The listing builds one solid part. Answer for the finished solid, in the listing's coordinates (mm). Face numbers are marked on the shaded views. A direction names the side the tool comes from. Give positions to 0.01 mm unless a question says otherwise; leave off trailing zeros. Order: outer loops, then holes, each group sorted by start corner. A loop starts at its lowest first (then second) coordinate and runs counter-clockwise, first axis right, second up.
```python
from build123d import *

# Parameters (mm, degrees)
BOSS_EXTRUDE1_DEPTH = 25.4
SKETCH3_R           = 4.05
CUT_EXTRUDE1_DEPTH  = 48.0377


with BuildPart() as part:
    # Sketch1 → Boss-Extrude1 (new body)
    with BuildSketch(Plane(origin=(0, 0, 0), x_dir=(0, 0, -1), z_dir=(1, 0, 0))):
        with BuildLine():
            Line((-1.764817843, 38.1), (-1.764817843, 34.67482934))
            ThreePointArc((-1.764817843, 34.67482934), (0, 22.225), (1.764817843, 34.67482934))
            Line((1.764817843, 34.67482934), (1.764817843, 38.1))
            Line((1.764817843, 38.1), (12.7, 38.1))
            Line((12.7, 38.1), (12.7, 9.46650416))
            Line((12.7, 9.46650416), (34.3377, 9.46650416))
            Line((34.3377, 9.46650416), (34.3377, -9.46650416))
            Line((34.3377, -9.46650416), (12.7, -9.46650416))
            Line((12.7, -9.46650416), (12.7, -38.1))
            Line((12.7, -38.1), (1.764817843, -38.1))
            Line((1.764817843, -38.1), (1.764817843, -31.585077082))
            ThreePointArc((1.764817843, -31.585077082), (0, -12.7), (-1.764817843, -31.585077082))
            Line((-1.764817843, -31.585077082), (-1.764817843, -38.1))
            Line((-1.764817843, -38.1), (-12.7, -38.1))
            Line((-12.7, -38.1), (-12.7, 38.1))
            Line((-12.7, 38.1), (-1.764817843, 38.1))
        make_face()
    extrude(amount=BOSS_EXTRUDE1_DEPTH)

    # Sketch3 → Cut-Extrude1 (cut, through all)
    with BuildSketch(Plane(origin=(0, 0, -34.3377), x_dir=(-1, 0, 0), z_dir=(0, 0, -1))):
        with Locations((-12.7, -3.002772529)):
            Circle(SKETCH3_R)
    extrude(amount=-CUT_EXTRUDE1_DEPTH, mode=Mode.SUBTRACT)


solid = part.part
```
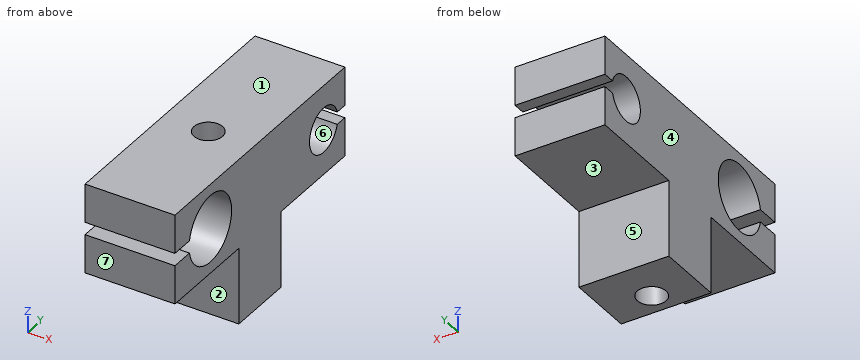
1) A tool of negligible diameter and unlimited length cuts with its end or side. For the marked faces 1, 2 and 3, from which of +Z, -Z, +X, -X, +Y, -Y can it reach the whole face along a straight path? Write none if from no direction.
Geometry says:
face 1: +Z, +X, -X, +Y, -Y
face 2: -Z, +X, -X, -Y
face 3: -Z, +X, -X, +Y
2) Find section B-B (z = -8). Write down the section's boundary in (x, y).
Geometry says:
outline: (0, -38.1) - (25.4, -38.1) - (25.4, -27.39) - (0, -27.39) - close; (0, -17.06) - (25.4, -17.06) - (25.4, 38.1) - (0, 38.1) - close; hole circle Ø8.1 at (12.7, -3)
3) For a pull along Y with two mould halves and no side action, classify the marked faces 4, 5, 6 and 7 as +Y half, -Y half, draft (parallel to the pull), parting line (faces both ways), or undercut.
Geometry says:
face 4: draft
face 5: +Y half
face 6: undercut
face 7: -Y half
4) Given P1, Ø7.5, axis at x = 12.5, y = 26, coming from the -Z side; P2, Ø12, axis at x = 18.5, z = -26.5, coming from the +Y side; P3, Ø11, axis at x = 18, z = -23.5, coming from the -Y side; P4, Ø11.5, axis at y = -22.225, z = 0, coming from the +X side, each flat-ended and moving along its own axis, determine where each tip first touches the part or whether it passes through.
Geometry says:
P1: stops at z = -12.7
P2: stops at y = 9.47
P3: stops at y = -9.47
P4: passes through
5) Find section C-C (y = -15.5). Write down the section's boundary in (x, z).
Geometry says:
outline: (0, -12.7) - (25.4, -12.7) - (25.4, -6.75) - (0, -6.75) - close; (0, 6.75) - (25.4, 6.75) - (25.4, 12.7) - (0, 12.7) - close
6) Straight lines are drawn through the part: probe 1 along Z at (x, y) = (11.5, -34); probe 2 along Y at (x, z) = (12.7, -17); probe 3 along Z at (x, y) = (9.25, 29.5). For each, find the intervals that lie inside material, in ascending order.
Geometry says:
probe 1: z = -12.7 to -1.76, 1.76 to 12.7
probe 2: y = -9.47 to -7.05, 1.05 to 9.47
probe 3: z = -12.7 to -6.28, 6.28 to 12.7
